Source: CAD feature listing. Evaluate the final solid. Frame: model axes, mm. Face numbers are marked on the shaded views. A direction names the side the tool comes from. Round coordinates to 2 decimals unless told otherwise and drop trailing zeros. Loops run counter-clockwise (first coordinate to the right, second up) from the corner with the lowest first, then second, coordinate; pieces in that order, holes last. Notation, with made-up numbers: M -11.5,-39.5 L 2.5,-39.5 A26 ccw 2.5,-19.5 Z; hole C -15,-10 d1. An arc over 180 degrees is marked long. Answer as a JSON object with one key per item and string values.
Autodesk Fusion 360 part; units mm, degrees
sketch "Sketch1" plane through (0, 0, 0) normal (0, 0, 1) x (1, 0, 0) in component "New Design"
  line L0 (-73, 36) -> (73, 36)
  line L1 (73, 36) -> (73, -36)
  line L2 (73, -36) -> (-73, -36)
  line L3 (-73, -36) -> (-73, 36)
  line L4 (-73, 36) -> (73, -36) construction
  line L5 (73, 36) -> (-73, -36) construction
  line L6 (-73, -36) -> (-1, -36)
  line L7 (-1, -36) -> (-1, 14)
  line L8 (-1, 14) -> (-73, 14)
  line L9 (-73, 14) -> (-73, -36)
  line L10 (23.0005, 12) -> (73, 11.9981)
  line L11 (23.0005, -12) -> (73, -11.9981)
  arc A0 (24.2094, 11.9389) -> (24.2094, -11.9389) centre (23, 0) ccw
  dimension "d1" = 146
  dimension "d2" = 72
  dimension "d3" = 72
  dimension "d4" = 50
  dimension "d5" = 24
  dimension "d6" = 50
extrude "Extrude1" add sketch "Sketch1" along normal blind 25 contours L0 L1 L2 L3 L7 L8 L10 L11 A0 | L2 L3 L6 L7 L8 L9 in component "New Design"
extrude "Extrude2" cut sketch "Sketch1" along normal blind 6 contours L2 L3 L6 L7 L8 L9 in component "New Design"
sketch "Sketch2" plane through (0, 0, 25) normal (0, 0, 1) x (-1, 0, 0) in component "New Design"
  arc A0 (-23.0005, -12) -> (-23.0005, 12) centre (-23, 0) ccw
  line L0 (-23.0005, -12) -> (-73, -11.9981)
  line L1 (-73, -11.9981) -> (-73, -36)
  line L2 (-73, -36) -> (73, -36)
  line L3 (73, -36) -> (73, 36)
  line L4 (73, 36) -> (-73, 36)
  line L5 (-73, 36) -> (-73, 11.9981)
  line L6 (-73, 11.9981) -> (-23.0005, 12)
  line L7 (73, -36) -> (37, -36)
  line L8 (37, -36) -> (37, 36)
  line L9 (37, 36) -> (73, 36)
  line L10 (73, 36) -> (73, -36)
  dimension "d11" = 36
extrude "Extrude3" add sketch "Sketch2" along normal blind 65 contours L2 L3 L4 L7 L8 L9 L10 in component "New Design"
sketch "Sketch3" plane through (-73, 0, 0) normal (-1, 0, 0) x (0, -1, 0) in component "New Design"
  line L0 (-14, 0) -> (-14, 6)
  line L1 (-14, 6) -> (36, 6)
  line L2 (36, 6) -> (36, 90)
  line L3 (36, 90) -> (-36, 90)
  line L4 (-36, 90) -> (-36, 0)
  line L5 (-36, 0) -> (-14, 0)
sketch "Sketch4" plane through (-73, 0, 45) normal (-1, 0, 0) x (0, -1, 0) in component "New Design"
  circle A0 centre (0, 3) radius 12
  circle A1 centre (0, 3) radius 30
  line L0 (-36, 45) -> (36, 45)
  line L1 (36, 45) -> (36, 21)
  line L2 (36, 21) -> (-36, 21)
  line L3 (-36, 21) -> (-36, 45)
  line L4 (36, -39) -> (-36, -39)
  line L5 (-36, -39) -> (-36, -15)
  line L6 (-36, -15) -> (36, -15)
  line L7 (36, -15) -> (36, -39)
  point P0 (0, -45)
  dimension "d14" = 24
  dimension "d15" = 60
  dimension "d16" = 48
  dimension "d17" = 24
  dimension "d18" = 24
extrude "Extrude4" cut sketch "Sketch4" against normal blind 100 contours A0 in component "New Design"
sketch "Sketch5" plane through (-73, 0, 45) normal (-1, 0, 0) x (0, -1, 0) in component "New Design"
  line L0 (-24, 21) -> (-36, 21)
  line L1 (-36, 21) -> (-36, -15)
  line L2 (-36, -15) -> (-24, -15)
  line L3 (24, 21) -> (36, 21)
  line L4 (36, 21) -> (36, -15)
  line L5 (36, -15) -> (24, -15)
extrude "Extrude5" cut sketch "Sketch4" against normal blind 12 contours A1 L2 L6 | A1 L2 | A1 L6 in component "New Design"
sketch "Sketch6" plane through (-73, 0, 0) normal (-1, 0, 0) x (0, -1, 0) in component "New Design"
  circle A0 centre (0, 48) radius 30
  line L0 (-14, 0) -> (-14, 6)
  line L1 (-14, 6) -> (36, 6)
  line L2 (36, 6) -> (36, 90)
  line L3 (36, 90) -> (-36, 90)
  line L4 (-36, 90) -> (-36, 0)
  line L5 (-36, 0) -> (-14, 0)
  line L6 (-22.3869, 67.9706) -> (-41.8695, 67.9706)
  line L7 (-41.8695, 67.9706) -> (-41.8695, 28.0294)
  line L8 (-41.8695, 28.0294) -> (-22.3869, 28.0294)
  line L9 (-22.3869, 28.0294) -> (-22.3869, 67.9706)
  line L10 (0, 90) -> (0, 18)
  line L11 (41.8695, 28.0294) -> (22.3869, 28.0294)
  line L12 (22.3869, 28.0294) -> (22.3869, 67.9706)
  line L13 (41.8695, 67.9706) -> (41.8695, 28.0294)
  line L14 (22.3869, 67.9706) -> (41.8695, 67.9706)
  dimension "d23" = 19.4825
extrude "Extrude6" cut sketch "Sketch6" against normal blind 12 contours A0 L2 L11 L14 | A0 L4 L6 L8 in component "New Design"
component "New Design" placed x (1, 0, 0) y (0, 1, 0) z (0, 0, 1) at (0, 0, 0)
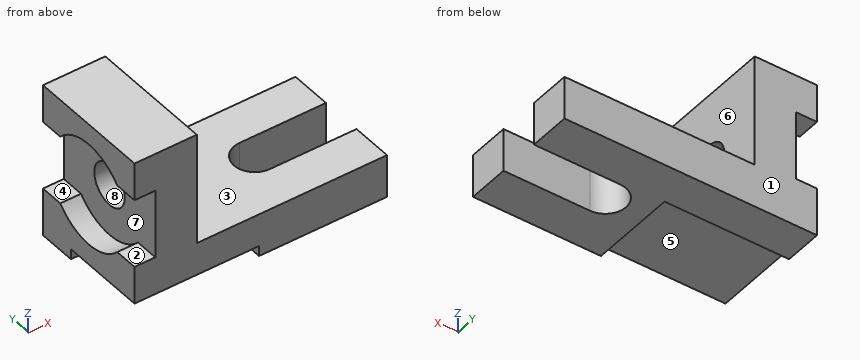
Item 1: Section B-B on z = 48. Return the cut outline in (x, y), then the cut area to 3 significant figures.
Answer sheet:
{"outline": "M -61,-36 L -37,-36 L -37,-12 L -61,-12 Z; M -61,12 L -37,12 L -37,36 L -61,36 Z", "area": "1,150 mm²"}
Item 2: Line query: probe 1 along Z at (x, y) = (-47.5, 0); probe 2 along Z at (x, y) = (41, -26); probe 3 along Z at (x, y) = (-42, -1.5). Output: solid intervals per line, ascending. Write a range as from..to.
Answer sheet:
{"probe 1": "z = 6..36, 60..90", "probe 2": "z = 0..25", "probe 3": "z = 6..36.09, 59.91..90"}
Item 3: Access query for the marked faces 4, 5, 6, 7 and 8. Directions: +Z, -Z, +X, -X, +Y, -Y. A direction counts if a zero-diameter tool reaches every point of the face in a straight line with its end or side. Return the directions, or none.
Answer sheet:
{"face 4": "-X, +Y, -Y", "face 5": "-Z, -X, -Y", "face 6": "+Z, +X, +Y, -Y", "face 7": "-X", "face 8": "+X, -X"}
Item 4: Pull-direction query (Z, two-part tool) for the marked faces 1, 2 and 3; classes: pulls with the +Z half, pulls with the -Z half, needs draft (parallel to the pull), parting line crosses it, or undercut.
Answer sheet:
{"face 1": "needs draft", "face 2": "undercut", "face 3": "pulls with the +Z half"}
Item 5: Contact query for flat-ended pins moving along their axis: pin 1 Ø5 at (y, z) = (-15, 58.5) entering from -X; pin 2 Ø21.5 at (x, y) = (13, 7) entering from +Z; pin 3 Ø3 at (y, z) = (-18, 3.5) entering from -X. Output: stop coordinate, or through.
Answer sheet:
{"pin 1": "stops at x = -61", "pin 2": "stops at z = 25", "pin 3": "stops at x = -1"}
Item 6: Section A-A on y = 0. Return the cut outline in (x, z).
Answer sheet:
{"outline": "M -73,6 L -1,6 L -1,0 L 11,0 L 11,25 L -37,25 L -37,36 L -61,36 L -61,18 L -73,18 Z; M -73,78 L -61,78 L -61,60 L -37,60 L -37,90 L -73,90 Z"}
Item 7: Section D-D on x = -3.5. Return the cut outline in (y, z), then the cut area to 3 significant figures.
Answer sheet:
{"outline": "M -36,6 L 14,6 L 14,0 L 36,0 L 36,25 L -36,25 Z", "area": "1,500 mm²"}
Item 8: Section C-C on x = -54.5. Return the cut outline in (y, z), then the cut area to 3 significant figures.
Answer sheet:
{"outline": "M -36,6 L 14,6 L 14,0 L 36,0 L 36,90 L -36,90 Z; hole C 0,48 d24", "area": "5,730 mm²"}
